Geometry check sheet. Reference: the model listing, model coordinates, mm. A direction names the side the tool comes from. Give positions to 0.01 mm unless a question says otherwise; leave off trailing zeros. Write each loop counter-clockwise with the first axis right and the second up, starting at its lowest first coordinate (ties: lowest second). Pieces come first, ordered by that corner, then holes. Notation, with made-up numbers: M 10,65 L 56,65 A19 cw 56,94 Z; hole C 82,20.5 d6. An arc over 180 degrees is marked long. Use one line per item in the form item = value. Start each with the question number.
```python
from build123d import *

# Parameters (mm, degrees)
SKETCH_2_W          = 46
SKETCH_2_H          = 36
SKETCH_2_R          = 1.65
EXTRUDE_1_DEPTH     = 3
SKETCH_3_W          = 3
SKETCH_3_H          = 36
EXTRUDE_2_DEPTH     = 13
CUT_EXTRUDE_1_DEPTH = 50
FILLET_1_R          = 2


with BuildPart() as part:
    # 草图2 → 凸台-拉伸1 (new body)
    with BuildSketch(Plane.XY):
        with Locations((23, 18)):
            Rectangle(SKETCH_2_W, SKETCH_2_H)
        with Locations((23, 18)):
            Circle(SKETCH_2_R, mode=Mode.SUBTRACT)
        with Locations((31, 18)):
            Circle(SKETCH_2_R, mode=Mode.SUBTRACT)
        with Locations((23, 26)):
            Circle(SKETCH_2_R, mode=Mode.SUBTRACT)
        with Locations((31, 26)):
            Circle(SKETCH_2_R, mode=Mode.SUBTRACT)
        with Locations((15, 26)):
            Circle(SKETCH_2_R, mode=Mode.SUBTRACT)
        with Locations((31, 10)):
            Circle(SKETCH_2_R, mode=Mode.SUBTRACT)
        with Locations((15, 18)):
            Circle(SKETCH_2_R, mode=Mode.SUBTRACT)
        with Locations((23, 10)):
            Circle(SKETCH_2_R, mode=Mode.SUBTRACT)
        with Locations((15, 10)):
            Circle(SKETCH_2_R, mode=Mode.SUBTRACT)
    extrude(amount=EXTRUDE_1_DEPTH)

    # 草图3 → 凸台-拉伸2 (add)
    with BuildSketch(Plane.XY.offset(3)):
        with Locations((1.5, 18)):
            Rectangle(SKETCH_3_W, SKETCH_3_H)
        with Locations((44.5, 18)):
            Rectangle(SKETCH_3_W, SKETCH_3_H)
    extrude(amount=EXTRUDE_2_DEPTH)

    # 草图4 → 切除-拉伸1 (cut)
    with BuildSketch(Plane(origin=(0, 0, 0), x_dir=(0, 0, -1), z_dir=(1, 0, 0))):
        with BuildLine():
            ThreePointArc((-9.35, 26), (-9.833273811, 27.166726189), (-11, 27.65))
            Line((-11, 27.65), (-11, 24.35))
            ThreePointArc((-11, 24.35), (-9.833273811, 24.833273811), (-9.35, 26))
        make_face()
        with BuildLine():
            Line((-11, 24.35), (-11, 27.65))
            ThreePointArc((-11, 27.65), (-12.65, 26), (-11, 24.35))
        make_face()
        with BuildLine():
            ThreePointArc((-11, 19.65), (-12.65, 18), (-11, 16.35))
            Line((-11, 16.35), (-11, 19.65))
        make_face()
        with BuildLine():
            Line((-11, 19.65), (-11, 16.35))
            ThreePointArc((-11, 16.35), (-9.833273811, 16.833273811), (-9.35, 18))
            ThreePointArc((-9.35, 18), (-9.833273811, 19.166726189), (-11, 19.65))
        make_face()
        with BuildLine():
            ThreePointArc((-11, 11.65), (-12.65, 10), (-11, 8.35))
            Line((-11, 8.35), (-11, 11.65))
        make_face()
        with BuildLine():
            Line((-11, 11.65), (-11, 8.35))
            ThreePointArc((-11, 8.35), (-9.833273811, 8.833273811), (-9.35, 10))
            ThreePointArc((-9.35, 10), (-9.833273811, 11.166726189), (-11, 11.65))
        make_face()
    extrude(amount=CUT_EXTRUDE_1_DEPTH, mode=Mode.SUBTRACT)

    # 圆角1
    fillet_1_edges = [part.edges().sort_by_distance(p)[0] for p in [
        (1.5, 36, 16),
        (1.5, 0, 16),
        (44.5, 0, 16),
        (44.5, 36, 16),
    ]]
    fillet(fillet_1_edges, radius=FILLET_1_R)


solid = part.part
```
(1) Sectioned sample at A-A, the plane z = 4.75. Record the boundary of the cut face in (x, y), plus the area to 3 significant figures.
(2) Depth check by flat-ended pin: pin 1 (6 mm diameter, centred on x = 7.5, z = 7.5, fed in from -Y); pin 2 (5.5 mm diameter, centred on x = 15, y = 10, fed in from +Z). Enter the tip coordinate at first touch or a pass-through.
(3) Sectioned sample at C-C, the plane y = 33.5. Record the boundary of the cut face in (x, z), plus the area to 3 significant figures.
(4) Draft check along Y on faces 1 (the cylindrical face through (16.524, 9.368, 1.479)), 2 (the flat face through (44, 18, 16)), 3 (the cylindrical face through (1.52, 0.6, 15.43)), 4 (the cylindrical face through (44.52, 35.43, 15.4)). Enter one of: released by +Y, released by -Y, zero draft, split by the parting line, or undercut.
(5) Sectioned sample at D-D, the plane z = 2.25. State how many separate pieces and enclosed holes the cut face has, plus the area to 3 significant figures.
(6) Sectioned sample at B-B, the plane x = 31. Record the boundary of the cut face in (y, z), plus the area to 3 significant figures.
(7) Tool access check on faces 5 (the cylindrical face through (15.89, 27.39, 1.48)), 6 (the flat face through (23, 14, 3)). Record the directions out of +Z, -Z, +X, -X, +Y, -Y that give a thin tool (end or side, any length) a straight path to the whole face; none if there is none.
(8) Thickness scan on probe 1 along Y at (x, z) = (23, 0.95); probe 2 along X at (y, z) = (16, 4.5); probe 3 along X at (y, z) = (24.5, 2). Record the ranges inside material, lowest first. Write a range as [from, to].
Numbers:
q1.outline = M 0,0 L 3,0 L 3,36 L 0,36 Z; M 43,0 L 46,0 L 46,36 L 43,36 Z
q1.area = 216 mm2
q2.pin_1 = through
q2.pin_2 = 3
q3.outline = M 0,0 L 46,0 L 46,16 L 43,16 L 43,3 L 3,3 L 3,16 L 0,16 Z
q3.area = 216 mm2
q4.face_1 = undercut
q4.face_2 = zero draft
q4.face_3 = released by -Y
q4.face_4 = released by +Y
q5.separate_pieces = 1
q5.enclosed_holes = 9
q5.area = 1,580 mm2
q6.outline = M 0,0 L 8.35,0 L 8.35,3 L 0,3 Z; M 11.65,0 L 16.35,0 L 16.35,3 L 11.65,3 Z; M 19.65,0 L 24.35,0 L 24.35,3 L 19.65,3 Z; M 27.65,0 L 36,0 L 36,3 L 27.65,3 Z
q6.area = 78.3 mm2
q7.face_5 = +Z, -Z
q7.face_6 = +Z, +Y, -Y
q8.probe_1 = [0, 8.35], [11.65, 16.35], [19.65, 24.35], [27.65, 36]
q8.probe_2 = [0, 3], [43, 46]
q8.probe_3 = [0, 14.31], [15.69, 22.31], [23.69, 30.31], [31.69, 46]
